Part model, mm, in its own coordinate system. A direction names the side the tool comes from. Give positions to 0.01 mm unless a question says otherwise; leave off trailing zeros. Order: outer loops, then holes, each group sorted by start corner. A loop starts at its lowest first (then second) coordinate and runs counter-clockwise, first axis right, second up. Notation, with made-up numbers: M 81,-31 L 92,-31 A35 ccw 92,1 Z; hole C 86.5,26.25 d8. An arc over 180 degrees is marked long. Answer as a JSON object with one key per item and string values.
from build123d import *

# Parameters (mm, degrees)
F0_R     = 12.6
F1_DEPTH = 10
F2_R     = 0.5


with BuildPart() as f1:
    # F0 (on Top) → F1 (new body)
    with BuildSketch(Plane.XY):
        with BuildLine():
            Line((42.497423, -38.607695), (15.155445, 8.75))
            ThreePointArc((15.155445, 8.75), (0, 17.5), (-15.155445, 8.75))
            Line((-15.155445, 8.75), (-42.497423, -38.607695))
            ThreePointArc((-42.497423, -38.607695), (-43.096825, -40.054781), (-43.30127, -41.607695))
            Line((-43.30127, -41.607695), (-43.30127, -50))
            Line((-43.30127, -50), (-33.30127, -50))
            Line((-33.30127, -50), (-33.30127, -40))
            Line((-33.30127, -40), (33.30127, -40))
            Line((33.30127, -40), (33.30127, -50))
            Line((33.30127, -50), (43.30127, -50))
            Line((43.30127, -50), (43.30127, -41.607695))
            ThreePointArc((43.30127, -41.607695), (43.096825, -40.054781), (42.497423, -38.607695))
        make_face()
        with BuildLine():
            Line((-19.529804, -18.668883), (19.132447, -18.668883))
            ThreePointArc((19.132447, -18.668883), (23.375088, -20.426242), (25.132447, -24.668883))
            Line((25.132447, -24.668883), (25.132447, -35.165567))
            Line((25.132447, -35.165567), (-25.529804, -35.165567))
            Line((-25.529804, -35.165567), (-25.529804, -24.668883))
            ThreePointArc((-25.529804, -24.668883), (-23.772444, -20.426242), (-19.529804, -18.668883))
        make_face(mode=Mode.SUBTRACT)
        Circle(F0_R, mode=Mode.SUBTRACT)
    extrude(amount=F1_DEPTH)

    # F2
    f2_edges = [f1.edges().sort_by_distance(p)[0] for p in [
        (28.826434, -14.928848, 10),
        (0, 17.5, 10),
        (-28.826434, -14.928848, 10),
        (-43.096825, -40.054781, 10),
        (-43.30127, -45.803848, 10),
        (-38.30127, -50, 10),
        (-33.30127, -45, 10),
        (0, -40, 10),
        (33.30127, -45, 10),
        (38.30127, -50, 10),
        (43.30127, -45.803848, 10),
        (43.096825, -40.054781, 10),
        (-0.198678, -18.668883, 10),
        (23.375088, -20.426242, 10),
        (25.132447, -29.917225, 10),
        (-0.198678, -35.165567, 10),
        (-25.529804, -29.917225, 10),
        (-23.772444, -20.426242, 10),
        (-12.6, 0, 10),
        (28.826434, -14.928848, 0),
        (0, 17.5, 0),
        (-28.826434, -14.928848, 0),
        (-43.096825, -40.054781, 0),
        (-43.30127, -45.803848, 0),
        (-38.30127, -50, 0),
        (-33.30127, -45, 0),
        (0, -40, 0),
        (33.30127, -45, 0),
        (38.30127, -50, 0),
        (43.30127, -45.803848, 0),
        (43.096825, -40.054781, 0),
        (-0.198678, -18.668883, 0),
        (23.375088, -20.426242, 0),
        (25.132447, -29.917225, 0),
        (-0.198678, -35.165567, 0),
        (-25.529804, -29.917225, 0),
        (-23.772444, -20.426242, 0),
        (-12.6, 0, 0),
    ]]
    fillet(f2_edges, radius=F2_R)


solid = f1.part
1. Which spindle directions (+Z, -Z, +X, -X, +Y, -Y) get a long thin tool onto all of the face, cutting with end or side? Do faces 1 (the cylindrical face through (43.102, -40.076, 4.937)), 2 (the cylindrical face through (23.33, -20.38, 4.94)). Say none if no direction does.
Worked answers:
{"face 1": "+Z, -Z, +X, +Y", "face 2": "+Z, -Z"}
2. Two-plate mould, pull along X, no slides. Class faces 3 (the flat face through (25.132, -30, 5)), 4 (the flat face through (29.018, -15.26, 4.937)), 5 (the flat face through (38, -50, 5)): +X half, -X half, draft (parallel to the pull), parting line (faces both ways), or undercut.
Worked answers:
{"face 3": "undercut", "face 4": "+X half", "face 5": "draft"}
3. Cut at A-A on x = 0. Give the cut face in (y, z), plus the area to 3 significant figures.
Worked answers:
{"outline": "M -40,0.5 A0.5 ccw -39.5,0 L -35.67,0 A0.5 ccw -35.17,0.5 L -35.17,9.5 A0.5 ccw -35.67,10 L -39.5,10 A0.5 ccw -40,9.5 Z; M -18.67,0.5 A0.5 ccw -18.17,0 L -13.1,0 A0.5 ccw -12.6,0.5 L -12.6,9.5 A0.5 ccw -13.1,10 L -18.17,10 A0.5 ccw -18.67,9.5 Z; M 12.6,0.5 A0.5 ccw 13.1,0 L 17,0 A0.5 ccw 17.5,0.5 L 17.5,9.5 A0.5 ccw 17,10 L 13.1,10 A0.5 ccw 12.6,9.5 Z", "area": "157 mm^2"}
4. Cut at B-B on z = 7.75. Give the cut face in (x, y), plus the area to 3 significant figures.
Worked answers:
{"outline": "M -43.3,-50 L -33.3,-50 L -33.3,-40 L 33.3,-40 L 33.3,-50 L 43.3,-50 L 43.3,-41.61 A6 ccw 42.5,-38.61 L 15.16,8.75 A17.5 ccw -15.16,8.75 L -42.5,-38.61 A6 ccw -43.3,-41.61 Z; hole M -25.53,-35.17 L 25.13,-35.17 L 25.13,-24.67 A6 ccw 19.13,-18.67 L -19.53,-18.67 A6 ccw -25.53,-24.67 Z; hole C 0,0 d25.2", "area": "1,920 mm^2"}
5. Probe line 1 along Y through (x, z) = (0, 6); line 2 along Y through (x, z) = (9, 4.75); line 3 along X through (y, z) = (-46.5, 8.5). List the from-to ranges inside material, lowest first.
Worked answers:
{"line 1": "y = -40 to -35.17, -18.67 to -12.6, 12.6 to 17.5", "line 2": "y = -40 to -35.17, -18.67 to -8.82, 8.82 to 15.01", "line 3": "x = -43.3 to -33.3, 33.3 to 43.3"}
6. Pin check, flat tips, straight feed: P1, Ø6, axis at x = -9.5, z = 5.5, coming from the -Y side; P2, Ø1.5, axis at y = -23.5, z = 4.5, coming from the +X side. Stop position of each tip, or through.
Worked answers:
{"P1": "stops at y = -40", "P2": "stops at x = 34.21"}
